Check sheet for the modelled part. Datum: model origin and axes. Units: mm. Round coordinates to 2 decimals unless told otherwise and drop trailing zeros. Write each loop counter-clockwise with the first axis right and the second up, starting at its lowest first coordinate (ties: lowest second). Pieces come first, ordered by that corner, then holes. Notation, with made-up numbers: (78.5, -18.75) - (134.5, -18.75) arc R37 ccw to (134.5, 19.25) - close; hole circle Ø2 at (42.5, 58). An arc over 180 degrees is marked (long way). Answer as a JSON object with one key per item and string values. Group by question number.
Item 1: Sectioned sample at A-A on y = 185.5. Record the boundary of the cut face in (x, z).
Item 2: Thickness scan on line 1 (X direction, y = 100, z = 2.75); line 2 (X direction, y = 181, z = 5.25); line 3 (Y direction, x = -1069, z = 3.25). Record the ranges inside material, lowest first.
Item 3: Gauge pin test, flat ends, axial feed: P1, Ø10, axis at y = 67.5, z = 4.5, coming from the -X side; P2, Ø4.5, axis at y = 277, z = 3.5, coming from the -X side; P3, Ø4, axis at x = -539, y = 29, coming from the -Z side; P4, Ø3, axis at y = 313.5, z = 4.5, coming from the +X side. Record the tip position at first contact, or that the pin passes through.
```python
from build123d import *

# Parameters (mm, degrees)
SKETCH_W        = 1404
SKETCH_H        = 390
PAD_DEPTH       = 18
SKETCH001_W     = 9
SKETCH001_H     = 390
POCKET_DEPTH    = 9
SKETCH002_W     = 18
SKETCH002_H     = 390
POCKET001_DEPTH = 8
POCKET003_DEPTH = 18.001
SKETCH005_W     = 480
SKETCH005_H     = 320
POCKET004_DEPTH = 4
SKETCH006_R     = 2.5
POCKET005_DEPTH = 10


with BuildPart() as part:
    # Sketch → Pad (new body)
    with BuildSketch(Plane.XY):
        with Locations((-702, 195)):
            Rectangle(SKETCH_W, SKETCH_H)
    extrude(amount=PAD_DEPTH)

    # Sketch001 → Pocket (cut)
    with BuildSketch(Plane.XY):
        with Locations((-4.5, 195)):
            Rectangle(SKETCH001_W, SKETCH001_H)
        with Locations((-1399.5, 195)):
            Rectangle(SKETCH001_W, SKETCH001_H)
    extrude(amount=POCKET_DEPTH, mode=Mode.SUBTRACT)

    # Sketch002 (on Face4 of Pocket) → Pocket001 (cut)
    with BuildSketch(Plane(origin=(0, 0, 0), x_dir=(1, 0, 0), z_dir=(0, 0, -1))):
        with Locations((-318, -195)):
            Rectangle(SKETCH002_W, SKETCH002_H)
    extrude(amount=-POCKET001_DEPTH, mode=Mode.SUBTRACT)

    # Sketch004 → Pocket003 (cut, through all)
    with BuildSketch(Plane(origin=(0, 0, 0), x_dir=(1, 0, 0), z_dir=(0, 0, -1))):
        with BuildLine():
            Line((-383.35, -350), (-829.65, -350))
            ThreePointArc((-836, -343.65), (-834.140128, -348.140128), (-829.65, -350))
            Line((-836, -56.35), (-836, -343.65))
            ThreePointArc((-829.65, -50), (-834.140128, -51.859872), (-836, -56.35))
            Line((-383.35, -50), (-829.65, -50))
            ThreePointArc((-377, -56.35), (-378.859872, -51.859872), (-383.35, -50))
            Line((-377, -343.65), (-377, -56.35))
            ThreePointArc((-383.35, -350), (-378.859872, -348.140128), (-377, -343.65))
        make_face()
        with BuildLine():
            Line((-886, -56.35), (-886, -343.65))
            ThreePointArc((-892.35, -350), (-887.859872, -348.140128), (-886, -343.65))
            Line((-892.35, -350), (-1338.65, -350))
            ThreePointArc((-1345, -343.65), (-1343.140128, -348.140128), (-1338.65, -350))
            Line((-1345, -343.65), (-1345, -56.35))
            ThreePointArc((-1338.65, -50), (-1343.140128, -51.859872), (-1345, -56.35))
            Line((-1338.65, -50), (-892.35, -50))
            ThreePointArc((-886, -56.35), (-887.859872, -51.859872), (-892.35, -50))
        make_face()
    extrude(amount=-POCKET003_DEPTH, mode=Mode.SUBTRACT)

    # Sketch005 (on Face4 of Pocket003) → Pocket004 (cut)
    with BuildSketch(Plane(origin=(0, 0, 0), x_dir=(1, 0, 0), z_dir=(0, 0, -1))):
        with Locations((-606, -200)):
            Rectangle(SKETCH005_W, SKETCH005_H)
        with Locations((-1116, -200)):
            Rectangle(SKETCH005_W, SKETCH005_H)
    extrude(amount=-POCKET004_DEPTH, mode=Mode.SUBTRACT)

    # Sketch006 (on Face4 of Pocket004) → Pocket005 (cut)
    with BuildSketch(Plane(origin=(0, 0, 0), x_dir=(1, 0, 0), z_dir=(0, 0, -1))):
        with Locations((-433, -29)):
            Circle(SKETCH006_R)
        with Locations((-539, -29)):
            Circle(SKETCH006_R)
        with Locations((-645, -29)):
            Circle(SKETCH006_R)
        with Locations((-751, -29)):
            Circle(SKETCH006_R)
        with Locations((-857, -29)):
            Circle(SKETCH006_R)
        with Locations((-963, -29)):
            Circle(SKETCH006_R)
        with Locations((-1069, -29)):
            Circle(SKETCH006_R)
        with Locations((-1175, -29)):
            Circle(SKETCH006_R)
        with Locations((-1281, -29)):
            Circle(SKETCH006_R)
        with Locations((-433, -371)):
            Circle(SKETCH006_R)
        with Locations((-539, -371)):
            Circle(SKETCH006_R)
        with Locations((-645, -371)):
            Circle(SKETCH006_R)
        with Locations((-751, -371)):
            Circle(SKETCH006_R)
        with Locations((-857, -371)):
            Circle(SKETCH006_R)
        with Locations((-963, -371)):
            Circle(SKETCH006_R)
        with Locations((-1069, -371)):
            Circle(SKETCH006_R)
        with Locations((-1175, -371)):
            Circle(SKETCH006_R)
        with Locations((-1281, -371)):
            Circle(SKETCH006_R)
    extrude(amount=-POCKET005_DEPTH, mode=Mode.SUBTRACT)


solid = part.part
```
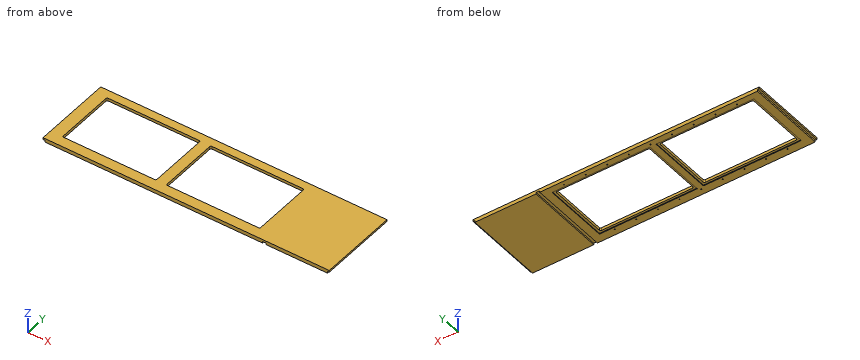
Completed:
{
 "1": {"outline": "(-1404, 9) - (-1395, 9) - (-1395, 0) - (-1356, 0) - (-1356, 4) - (-1345, 4) - (-1345, 18) - (-1404, 18) - close; (-886, 4) - (-876, 4) - (-876, 0) - (-846, 0) - (-846, 4) - (-836, 4) - (-836, 18) - (-886, 18) - close; (-377, 4) - (-366, 4) - (-366, 0) - (-327, 0) - (-327, 8) - (-309, 8) - (-309, 0) - (-9, 0) - (-9, 9) - (0, 9) - (0, 18) - (-377, 18) - close"},
 "2": {"line 1": "-1395 to -1356, -876 to -846, -366 to -327, -309 to -9", "line 2": "-1395 to -1345, -886 to -836, -377 to -327, -309 to -9", "line 3": "0 to 26.5, 31.5 to 40, 360 to 368.5, 373.5 to 390"},
 "3": {"P1": "x = -1404", "P2": "x = -1395", "P3": "z = 10", "P4": "x = -9"}
}
